```python
from build123d import *

# Parameters (mm, degrees)
SKETCH1_W           = 65
SKETCH1_H           = 40
BOSS_EXTRUDE1_DEPTH = 17
SKETCH2_W           = 11.5
SKETCH2_H           = 40
BOSS_EXTRUDE2_DEPTH = 53
FILLET1_R           = 20
CHAMFER1_SIZE       = 5
SKETCH3_R           = 5
CUT_EXTRUDE1_DEPTH  = 10
SKETCH4_R           = 5
BOSS_EXTRUDE3_DEPTH = 10


with BuildPart() as part:
    # Sketch1 → Boss-Extrude1 (new body)
    with BuildSketch(Plane.XY):
        with Locations((32.5, 20)):
            Rectangle(SKETCH1_W, SKETCH1_H)
    extrude(amount=BOSS_EXTRUDE1_DEPTH)

    # Sketch2 → Boss-Extrude2 (add)
    with BuildSketch(Plane(origin=(0, 0, 0), x_dir=(-1, 0, 0), z_dir=(0, 0, -1))):
        with Locations((-5.75, 20)):
            Rectangle(SKETCH2_W, SKETCH2_H)
        with Locations((-59.25, 20)):
            Rectangle(SKETCH2_W, SKETCH2_H)
    extrude(amount=BOSS_EXTRUDE2_DEPTH)

    # Fillet1
    fillet1_edges = [part.edges().sort_by_distance(p)[0] for p in [
        (59.25, 40, -53),
        (5.75, 40, -53),
        (59.25, 0, -53),
        (5.75, 0, -53),
    ]]
    fillet(fillet1_edges, radius=FILLET1_R - 0.0001)  # a hair under: the kernel refuses the full size

    # Chamfer1
    chamfer1_edges = [part.edges().sort_by_distance(p)[0] for p in [
        (65, 5.857835087, -47.142164913),
        (65, 34.142164913, -47.142164913),
        (0, 5.857835087, -47.142164913),
        (0, 34.142164913, -47.142164913),
        (0, 0, -8.00005),
        (65, 0, -8.00005),
        (65, 40, -8.00005),
        (0, 40, -8.00005),
    ]]
    chamfer(chamfer1_edges, length=CHAMFER1_SIZE)

    # Sketch3 → Cut-Extrude1 (cut)
    with BuildSketch(Plane.XY.offset(17)):
        with Locations((32.5, 20)):
            Circle(SKETCH3_R)
    extrude(amount=-CUT_EXTRUDE1_DEPTH, mode=Mode.SUBTRACT)

    # Sketch4 → Boss-Extrude3 (add)
    with BuildSketch(Plane(origin=(11.5, 0, 0), x_dir=(0, 0, -1), z_dir=(1, 0, 0))):
        with Locations(Location((33, 20, 0), (0, 0, 270))):
            Circle(SKETCH4_R)
    extrude(amount=BOSS_EXTRUDE3_DEPTH)


solid = part.part
```
Could you check a few things on this model? Use its own coordinates, in mm. A direction names the side the tool comes from. Coordinates: 2 decimals unless noted, no trailing zeros. Order: outer loops, then holes, each group sorted by start corner. A loop starts at its lowest first (then second) coordinate and runs counter-clockwise, first axis right, second up. Notation, with made-up numbers: M 40.25,3 L 95.25,3 A14 ccw 95.25,15 Z; hole C 56.5,13.5 d2. An arc over 180 degrees is marked long. Use a Markdown table: item, result. Add a question column.
Q1. I want a section at A-A on x = 32.5. List the corners of the cut face in (y, z) for me, then the cut area to 3 significant figures.
Q2. I want a section at C-C on x = 40. List the corners of the cut face in (y, z) for me.
Q3. We'd pull the mould along X, two halves only. Please class faces 4 (the cylindrical face through (8.204, 33.986, -47.297)), 5 (the flat face through (65, 20, -16)), 6 (the flat face through (21.5, 20, -33)): pulls with the +X half, pulls with the -X half, needs draft (parallel to the pull), parting line crosses it, or undercut.
Q4. I'm going to push a flat-ended pin straight in: pin 1 (20 mm diameter, centred on x = 42.5, y = 11, fed in from -Z). Where does the tip first touch, or does it pass through?
Q5. Which directions (+Z, -Z, +X, -X, +Y, -Y) give clear straight access to the entire face, cutting with the end or side of a thin tool? Please do faces 1 (the flat face through (63, 37, -8)), 2 (the cylindrical face through (28.5, 17, 12.1)), 3 (the cylindrical face through (16, 25, -33)).
Q6. If I drill on L1, parallel to X at y = 10.5, z = -26; L2, parallel to Y at x = 32.5, z = 13.5; L3, parallel to Z at x = 44.5, y = 32, over which ranges is the centre line in solid material (lowest first)?
Checked values:
| question | item | result |
|---|---|---|
| 1 | outline | M 0,0 L 40,0 L 40,17 L 25,17 L 25,7 L 15,7 L 15,17 L 0,17 Z |
| 1 | area | 580 mm² |
| 2 | outline | M 0,0 L 40,0 L 40,17 L 0,17 Z |
| 3 | face 4 | needs draft |
| 3 | face 5 | pulls with the +X half |
| 3 | face 6 | undercut |
| 4 | pin 1 | z = 0 |
| 5 | face 1 | +Z, -Z, +X, +Y |
| 5 | face 2 | +Z |
| 5 | face 3 | none |
| 6 | L1 | 0 to 11.5, 53.5 to 65 |
| 6 | L2 | 0 to 15, 25 to 40 |
| 6 | L3 | 0 to 17 |
